Build history of the part. All positions in model axes, mm. Coordinates: 2 decimals unless noted, no trailing zeros. Loops run counter-clockwise (first coordinate to the right, second up) from the corner with the lowest first, then second, coordinate; pieces in that order, holes last.
(1) Slice it at A-A (z = -17). Give the cut face in (x, y).
(2) Slice it at D-D (z = -65.5). Give the cut face in (x, y).
(3) Flat gauge pins, fed straight in: P1, Ø0.5, axis at y = -0.5, z = 17.5, coming from the -X side; P2, Ø1, axis at x = 78, z = 86, coming from the +Y side. Where does each tip first touch, or does it go through?
(4) Slice it at B-B (x = 19). Give the cut face in (y, z), and give its area (3 significant figures).
(5) Two-plate mould, pull along Z, no slides. Class faces 1 (the face through (87.6, -0.5, 123.4)), 2 (the face through (87.4, -0.5, 93.4)), 3 (the face through (102.185, -0.493, 43.412)), 4 (the face through (-87.6, -0.5, 93.6)): pulls with the +Z half, pulls with the -Z half, needs draft (parallel to the pull), parting line crosses it, or undercut.
(6) Slice it at C-C (y = -0.65). Give the cut face in (x, z).
(7) Wall check: L1, parallel to Z at x = -17, y = -0.4; L2, parallel to X at y = -0.45, z = -9.5; L3, parallel to X at y = -0.55, z = -32. Give the ranges that are in metal, low to high.
from build123d import *

# Parameters (mm, degrees)
F0_W     = 104
F0_H     = 80
F0_W_2   = 160
F0_H_2   = 45
F1_DEPTH = 1


with BuildPart() as f1:
    # F0 (on Front) → F1 (new body)
    with BuildSketch(Plane.XZ):
        Polygon((-80, 86), (-80, 2), (-80, -86), (-1.5, -86), (4.5, -86), (80, -86), (80, 2), (80, 86), align=None)
        with Locations((0, 17.5)):
            Rectangle(F0_W, F0_H, mode=Mode.SUBTRACT)
        Polygon((102.5, 86), (80, 86), (80, 2), (125, 86), align=None)
        with Locations((0, 108.5)):
            Rectangle(F0_W_2, F0_H_2)
        Polygon((-95, 101), (-80, 86), (-80, 131), (-95, 116), align=None)
        Polygon((-80, 86), (-125, 86), (-80, 2), align=None)
        Polygon((80, 131), (80, 86), (95, 101), (95, 116), align=None)
    extrude(amount=F1_DEPTH)


solid = f1.part
Response values:
1. outline: (-80, -1) - (-52, -1) - (-52, 0) - (-80, 0) - close; (52, -1) - (80, -1) - (80, 0) - (52, 0) - close
2. outline: (-80, -1) - (80, -1) - (80, 0) - (-80, 0) - close
3. P1: stops at x = -88.44
3. P2: stops at y = 0
4. outline: (-1, -86) - (0, -86) - (0, -22.5) - (-1, -22.5) - close; (-1, 57.5) - (0, 57.5) - (0, 131) - (-1, 131) - close
4. area: 137 mm2
5. face 1: pulls with the +Z half
5. face 2: undercut
5. face 3: pulls with the -Z half
5. face 4: undercut
6. outline: (-125, 86) - (-80, 2) - (-80, -86) - (80, -86) - (80, 2) - (125, 86) - (80, 86) - (95, 101) - (95, 116) - (80, 131) - (-80, 131) - (-95, 116) - (-95, 101) - (-80, 86) - close; hole (-52, -22.5) - (52, -22.5) - (52, 57.5) - (-52, 57.5) - close
7. L1: z = -86 to -22.5, 57.5 to 131
7. L2: x = -80 to -52, 52 to 80
7. L3: x = -80 to 80
